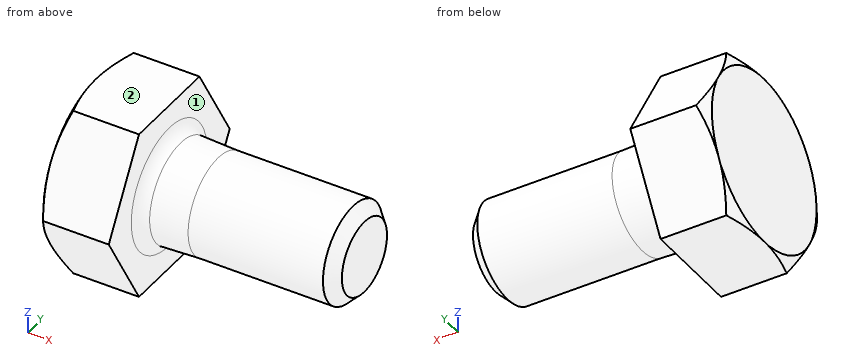
Autodesk Inventor part; units mm, degrees
ref_plane "Work Plane1" through (1.525, 0, 0) normal (0, 0, 1) x (1, 0, 0)
ref_plane "YZ Plane" through (0, 0, 0) normal (1, 0, 0) x (0, 1, 0)
ref_plane "XZ Plane" through (0, 0, 0) normal (0, 1, 0) x (-1, 0, 0)
sketch "Sketch1" plane through (0, 0, 0) normal (0, 0, 1) x (1, 0, 0)
  line L0 (0, 5.5626) -> (0, 3.302)
  line L1 (3.175, 3.175) -> (12.7, 3.175)
  line L2 (12.7, 3.175) -> (12.7, 0)
  line L3 (12.7, 0) -> (-0.0001, 0)
  line L4 (-2.5401, 0) -> (15.24, 0)
  line L5 (-0.0001, 0) -> (-0.0001, 5.5626)
  line L6 (-0.0001, 5.5626) -> (0, 5.5626)
  line L7 (3.175, 3.175) -> (0.0019, 3.302)
  line L8 (0.0019, 3.302) -> (0, 3.302)
  line L9 (0, -1.1125) -> (0, 6.6751)
  dimension "d0" = 12.7
  dimension "d1" = 9.525
  dimension "d2" = 6.35
  dimension "d9" = 0.0001
  dimension "d10" = 11.1252
  dimension "d13" = 3.1731
  dimension "d14" = 6.604
revolve "Body" add sketch "Sketch1" angle 360 about axis through (12.7, 0, 0) along (-1, 0, 0)
sketch "Sketch2" plane through (-0.0001, 0, 0) normal (-1, 0, 0) x (0, 0, 1)
  line L0 (0, 6.4231) -> (5.5626, 3.2116)
  line L1 (5.5626, 3.2116) -> (5.5626, -3.2116)
  line L2 (5.5626, -3.2116) -> (0, -6.4231)
  line L3 (0, -6.4231) -> (-5.5626, -3.2116)
  line L4 (-5.5626, -3.2116) -> (-5.5626, 3.2116)
  line L5 (-5.5626, 3.2116) -> (0, 6.4231)
  point P0 (0, 0)
  point P1 (0, 0)
  dimension "d11" = 11.1252
extrude "Head" add sketch "Sketch2" along normal blind 4.7752
sketch "Sketch4" plane through (0, 0, 0) normal (0, 0, 1) x (1, 0, 0)
  line L0 (-4.7753, 5.5626) -> (-4.7753, 6.4231)
  line L1 (-4.7753, 6.4231) -> (-4.2785, 6.4231)
  line L2 (-4.2785, 6.4231) -> (-4.7753, 5.5626)
  line L3 (-5.7303, 0) -> (0.9549, 0)
  line L4 (-0.0001, 6.4231) -> (-4.7753, 6.4231)
  line L5 (-4.7753, 3.2116) -> (-4.7753, 6.4231)
  dimension "d5" = 30
  dimension "d19" = 11.1252
revolve "Chamfer1" cut sketch "Sketch4" angle 360 about axis through (-10, 0, 0) along (1, 0, 0)
thread "Thread"
chamfer "Chamfer2" distance 0.7791 distance2 0.7553 1 edges at (12.7, -3.175, 0) measured on face at (12.7, 1.0276, -1.1503)
ref_plane "Work Plane1" through (1.525, 0, 0) normal (0, 0, 1) x (1, 0, 0)
fillet "Fillet2" radius 0.762 1 edges at (0.0019, -3.302, 0)
equation "\"d0\" = NLG"
equation "\"d1\" = GEL"
equation "\"d2\" = GD"
equation "\"d10\" = SD2"
equation "\"d14\" = BDM"
equation "\"d11\" = SW"
equation "\"d3\" = KOH - SD"
equation "\"d5\" = ANG1"
equation "\"d19\" = SW0"
equation "\"d63\" = R"
equation "\"d15\" = GEL"
equation "\"d6\" = -0.5 * SPD + 0.5 * GD"
equation "\"NLG\" = 12.7"
equation "\"GD\" = NND"
equation "\"BDM\" = 6.604"
equation "\"KOH\" = 4.7752"
equation "\"GEL\" = 9.525"
equation "\"SW\" = 11.1252"
equation "\"SW0\" = SW"
equation "\"SPD\" = GD1"
equation "\"SD2\" = SW"
equation "\"SD\" = 0"
equation "\"ANG1\" = 30deg"
equation "\"GAL\" = 3.173"
equation "\"GUL\" = 0.238 * GAL"
equation "\"R\" = 0.762"
equation "\"d62\" = -NLG - SD + GUL"
equation "\"GD1\" = 4.79184"
equation "\"THREADDIA\" = 6.35"
equation "\"TOA\" = 30deg"
equation "\"NND\" = 6.35"
equation "\"E0\" = 1.155 * SW"
properties part number "ANSI/ASME B18.2.1 - 1/4-20 UNC - 0.5" material "Steel, Mild"
Geometry check sheet. Reference: the model listing, model coordinates, mm. Face numbers are marked on the shaded views. A direction names the side the tool comes from. Give positions to 0.01 mm unless a question says otherwise; leave off trailing zeros. Loops run counter-clockwise (first coordinate to the right, second up) from the corner with the lowest first, then second, coordinate; pieces in that order, holes last.
(1) Section check A-A on x = -3.5. Record the cut outline in (y, z), then the cut area to 3 significant figures.
From the geometry:
outline: (-6.42, 0) - (-3.21, -5.56) - (3.21, -5.56) - (6.42, 0) - (3.21, 5.56) - (-3.21, 5.56) - close
area: 107 mm2
(2) Section check B-B on x = 4.5. Record the cut outline in (y, z) (3 decimals).
From the geometry:
outline: circle Ø6.35 at (0, 0)
(3) Thickness scan on L1, parallel to X at y = 4, z = -3.75; L2, parallel to Y at x = 2.25, z = 0.5; L3, parallel to Z at x = -2.75, y = -4.75. Record the ranges inside material, lowest first.
From the geometry:
L1: x = -4.78 to 0
L2: y = -3.17 to 3.17
L3: z = -2.9 to 2.9
(4) Set-up check for the marked faces 1 and 2: record each of +Z, -Z, +X, -X, +Y, -Y from which the full face is reachable in a straight line by a thin tool's end or side.
From the geometry:
face 1: +X
face 2: +Z, +X, -X, +Y, -Y
(5) Depth check by flat-ended pin: pin 1 Ø6 at (x, z) = (7.5, 0) entering from +Y (3 decimals); pin 2 Ø1 at (y, z) = (-0.5, -4) entering from +X; pin 3 Ø4 at (x, z) = (-2, 1) entering from -Y. Enter the tip coordinate at first touch or a pass-through.
From the geometry:
pin 1: stops at y = 3.175
pin 2: stops at x = 0.19
pin 3: stops at y = -6.42
(6) Section check C-C on x = 1.75. Record the cut outline in (y, z), then the cut area to 3 significant figures.
From the geometry:
outline: circle Ø6.46 at (0, 0)
area: 32.8 mm2
